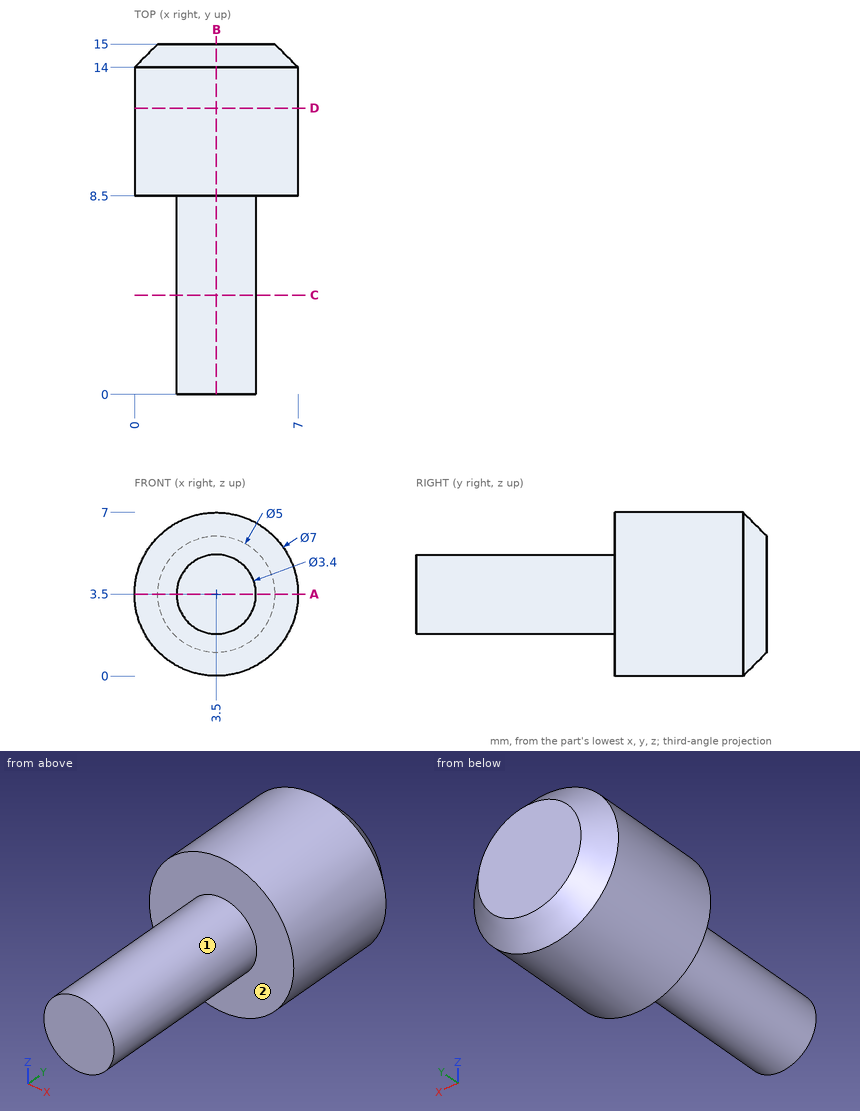
Source: three-view drawing plus pictorial views. Frame: mm from the lowest corner of the part. Coordinates: 2 decimals unless noted, no trailing zeros. Loops run counter-clockwise (first coordinate to the right, second up) from the corner with the lowest first, then second, coordinate; pieces in that order, holes last. Notation, with made-up numbers: (37, 58.5) - (69, 58.5) arc R26 cw to (69, 92.5) - close; hole circle Ø4 at (54, 10). An arc over 180 degrees is marked (long way). Answer in a Markdown table with one row per item. Add a question column.
Item 1: Section query B-B on x = 3.5. Return the cut outline in (y, z).
Item 2: Section query A-A on z = 3.5. Return the cut outline in (x, y).
Item 3: Line query: line 1 along Y through (x, z) = (4.5, 1.5); line 2 along X through (y, z) = (10.5, 4.5); line 3 along Y through (x, z) = (5.75, 1.5). Output: solid intervals per line, ascending. Write a range as [from, to].
Item 4: Section query D-D on y = 12.25. Return the cut outline in (x, z), then the cut area to 3 significant figures.
Item 5: Contact query for flat-ended pins moving along their axis: P1, Ø1, axis at y = 6.5, z = 5, coming from the +X side; P2, Ø1.5, axis at x = 5.5, y = 10.5, coming from the +Z side. Output: stop coordinate, or through.
Item 6: Section query C-C on y = 4.25. Return the cut outline in (x, z).
Item 7: Mould query, pull axis Z, two halves, no side actions, for the marked faces 1 and 2. Classes: released by +Z, released by -Z, zero draft, split by the parting line, or undercut.
Recorded:
| question | item | result |
|---|---|---|
| 1 | outline | (0, 1.8) - (8.5, 1.8) - (8.5, 0) - (14, 0) - (15, 1) - (15, 6) - (14, 7) - (8.5, 7) - (8.5, 5.2) - (0, 5.2) - close |
| 2 | outline | (0, 8.5) - (1.8, 8.5) - (1.8, 0) - (5.2, 0) - (5.2, 8.5) - (7, 8.5) - (7, 14) - (6, 15) - (1, 15) - (0, 14) - close |
| 3 | line 1 | [8.5, 15] |
| 3 | line 2 | [0.15, 6.85] |
| 3 | line 3 | [8.5, 14.49] |
| 4 | outline | circle Ø7 at (3.5, 3.5) |
| 4 | area | 38.5 mm^2 |
| 5 | P1 | x = 4.87 |
| 5 | P2 | z = 6.77 |
| 6 | outline | circle Ø3.4 at (3.5, 3.5) |
| 7 | face 1 | split by the parting line |
| 7 | face 2 | zero draft |
